Read the model definition and answer for the solid it produces. Units are mm, in the model's axes. A direction names the side the tool comes from. Coordinates: 2 decimals unless noted, no trailing zeros. Order: outer loops, then holes, each group sorted by start corner. A loop starts at its lowest first (then second) coordinate and runs counter-clockwise, first axis right, second up. Notation, with made-up numbers: (64.5, 21.25) -> (95.5, 21.25) arc R10 cw to (95.5, 35.25) -> close; hole circle Ø5 at (64.5, -34). An arc over 180 degrees is marked (long way). Answer in a Markdown table with one row per item.
from build123d import *

# Parameters (mm, degrees)
F1_DEPTH  = 6
F2_T      = -4
F3_DEPTH  = 25.4
F4_W      = 10.761987894
F4_H      = 6
F4_H_2    = 27.5
F5_DEPTH  = 4
F6_W      = 10.761987894
F6_H      = 6
F6_H_2    = 27.5
F7_DEPTH  = 4
F9_DEPTH  = 50
F10_DEPTH = 50
F11_DEPTH = 50
F12_DEPTH = 1
F13_DEPTH = 1
F14_DEPTH = 1
F15_DEPTH = 1
F18_DEPTH = 4
F20_DEPTH = 9
F21_R     = 1.5
F22_DEPTH = 7
F23_R     = 1.5
F24_DEPTH = 7
F25_R     = 1.5
F26_DEPTH = 7
F27_R     = 1.5
F28_DEPTH = 7
F29_R     = 7.5
F30_DEPTH = 25.4


with BuildPart() as f1:
    # F0 (on Top) → F1 (new body)
    with BuildSketch(Plane.XY):
        with BuildLine():
            Line((6.0000014261, 20.4372135154), (1.4261e-06, 20.4372135154))
            Line((1.4261e-06, 20.4372135154), (-5.9999985739, 20.4372135154))
            ThreePointArc((-5.9999985739, 20.4372135154), (-14.7648216341, 15.2020365756), (-19.9999985739, 6.4372135154))
            Line((-19.9999985739, 6.4372135154), (-19.9999985739, 0.4372135154))
            Line((-19.9999985739, 0.4372135154), (-19.9999985739, -5.5627864846))
            ThreePointArc((-19.9999985739, -5.5627864846), (-14.7648216341, -14.3276095448), (-5.9999985739, -19.5627864846))
            Line((-5.9999985739, -19.5627864846), (1.4261e-06, -19.5627864846))
            Line((1.4261e-06, -19.5627864846), (6.0000014261, -19.5627864846))
            ThreePointArc((6.0000014261, -19.5627864846), (14.7648244863, -14.3276095448), (20.0000014261, -5.5627864846))
            Line((20.0000014261, -5.5627864846), (20.0000014261, 6.4372135154))
            ThreePointArc((20.0000014261, 6.4372135154), (14.7648244863, 15.2020365756), (6.0000014261, 20.4372135154))
        make_face()
    extrude(amount=F1_DEPTH)

    # F2
    f2_openings = [f1.faces().sort_by_distance(p)[0] for p in [
        (1e-06, 0.437214, 6),
    ]]
    offset(amount=F2_T, openings=f2_openings)

    # F3 (cut): a face of the model
    f3_faces = [f1.faces().sort_by_distance(p)[0] for p in [
        (1.4261e-06, 0.4372135154, 4),
    ]]
    extrude(f3_faces, amount=-F3_DEPTH, mode=Mode.SUBTRACT)

    # F4 (on face) → F5 (join)
    with BuildSketch(Plane(origin=(16.0000014261, 0, 0), x_dir=(0, -1, 0), z_dir=(-1, 0, 0))):
        with Locations((-0.4372135154, 3)):
            Rectangle(F4_W, F4_H)
        with Locations((-0.4372135154, 19.75)):
            Rectangle(F4_W, F4_H_2)
    extrude(amount=-F5_DEPTH)

    # F6 (on face) → F7 (join)
    with BuildSketch(Plane.YZ.offset(-15.9999985739)):
        with Locations((0.4372135154, 3)):
            Rectangle(F6_W, F6_H)
        with Locations((0.4372135154, 19.75)):
            Rectangle(F6_W, F6_H_2)
    extrude(amount=-F7_DEPTH)

    # F8 (on face) → F9 (cut)
    with BuildSketch(Plane(origin=(-19.9999985739, 0, 0), x_dir=(0, -1, 0), z_dir=(-1, 0, 0))):
        with BuildLine():
            Line((-5.8182074624, 33.5), (-5.8182074624, 28.852354537))
            ThreePointArc((-5.8182074624, 28.852354537), (-3.9923402433, 32.177236302), (-0.4372135154, 33.5))
            Line((-0.4372135154, 33.5), (-5.8182074624, 33.5))
        make_face()
    extrude(amount=-F9_DEPTH, mode=Mode.SUBTRACT)

    # F8 (on face) → F10 (cut)
    with BuildSketch(Plane(origin=(-19.9999985739, 0, 0), x_dir=(0, -1, 0), z_dir=(-1, 0, 0))):
        with BuildLine():
            ThreePointArc((-0.4372135154, 33.5), (3.1179132125, 32.177236302), (4.9437804316, 28.852354537))
            Line((4.9437804316, 28.852354537), (4.9437804316, 33.5))
            Line((4.9437804316, 33.5), (-0.4372135154, 33.5))
        make_face()
    extrude(amount=-F10_DEPTH, mode=Mode.SUBTRACT)

    # F8 (on face) → F11 (cut)
    with BuildSketch(Plane(origin=(-19.9999985739, 0, 0), x_dir=(0, -1, 0), z_dir=(-1, 0, 0))):
        with BuildLine():
            ThreePointArc((3.8905718212, 24.7670060502), (4.0195248668, 25.3775186809), (4.0627864846, 26))
            ThreePointArc((4.0627864846, 26), (-1.0596948345, 30.4567383822), (-4.764998852, 24.7670060502))
            ThreePointArc((-4.764998852, 24.7670060502), (-0.4372135154, 21.5), (3.8905718212, 24.7670060502))
        make_face()
    extrude(amount=-F11_DEPTH, mode=Mode.SUBTRACT)

    # F12 (add): a face of the model
    f12_faces = [f1.faces().sort_by_distance(p)[0] for p in [
        (-17.9999985739, 5.8182074624, 17.4261772685),
    ]]
    extrude(f12_faces, amount=F12_DEPTH)

    # F13 (add): a face of the model
    f13_faces = [f1.faces().sort_by_distance(p)[0] for p in [
        (-17.9999985739, -4.9437804316, 17.4261772685),
    ]]
    extrude(f13_faces, amount=F13_DEPTH)

    # F14 (add): a face of the model
    f14_faces = [f1.faces().sort_by_distance(p)[0] for p in [
        (18.0000014261, 5.8182074624, 17.4261772685),
    ]]
    extrude(f14_faces, amount=F14_DEPTH)

    # F15 (add): a face of the model
    f15_faces = [f1.faces().sort_by_distance(p)[0] for p in [
        (18.0000014261, -4.9437804316, 17.4261772685),
    ]]
    extrude(f15_faces, amount=F15_DEPTH)

    # F17 (on face) → F18 (join)
    with BuildSketch(Plane(origin=(0, 0, 0), x_dir=(1, 0, 0), z_dir=(0, 0, -1))):
        with BuildLine():
            Line((1.4261e-06, 15.5627864846), (1.4261e-06, -0.4372135154))
            Line((1.4261e-06, -0.4372135154), (16.0000014261, -0.4372135154))
            Line((16.0000014261, -0.4372135154), (16.0000014261, 4.9437804316))
            ThreePointArc((16.0000014261, 4.9437804316), (11.9363973616, 11.4991824201), (5.3809953731, 15.5627864846))
            Line((5.3809953731, 15.5627864846), (1.4261e-06, 15.5627864846))
        make_face()
        with BuildLine():
            Line((-15.9999985739, 4.9437804316), (-15.9999985739, -0.4372135154))
            Line((-15.9999985739, -0.4372135154), (1.4261e-06, -0.4372135154))
            Line((1.4261e-06, -0.4372135154), (1.4261e-06, 15.5627864846))
            Line((1.4261e-06, 15.5627864846), (-5.3809925209, 15.5627864846))
            ThreePointArc((-5.3809925209, 15.5627864846), (-11.9363945094, 11.4991824201), (-15.9999985739, 4.9437804316))
        make_face()
        with BuildLine():
            Line((1.4261e-06, -0.4372135154), (-15.9999985739, -0.4372135154))
            Line((-15.9999985739, -0.4372135154), (-15.9999985739, -5.8182074624))
            ThreePointArc((-15.9999985739, -5.8182074624), (-11.9363945094, -12.3736094509), (-5.3809925209, -16.4372135154))
            Line((-5.3809925209, -16.4372135154), (1.4261e-06, -16.4372135154))
            Line((1.4261e-06, -16.4372135154), (1.4261e-06, -0.4372135154))
        make_face()
        with BuildLine():
            Line((16.0000014261, -0.4372135154), (1.4261e-06, -0.4372135154))
            Line((1.4261e-06, -0.4372135154), (1.4261e-06, -16.4372135154))
            Line((1.4261e-06, -16.4372135154), (5.3809953731, -16.4372135154))
            ThreePointArc((5.3809953731, -16.4372135154), (11.9363973616, -12.3736094509), (16.0000014261, -5.8182074624))
            Line((16.0000014261, -5.8182074624), (16.0000014261, -0.4372135154))
        make_face()
    extrude(amount=-F18_DEPTH)

    # F19 (on face) → F20 (join)
    with BuildSketch(Plane(origin=(0, 0, 0), x_dir=(1, 0, 0), z_dir=(0, 0, -1))):
        with BuildLine():
            Line((6, 31), (0, 31))
            Line((0, 31), (-6, 31))
            ThreePointArc((-6, 31), (-22.3271135618, 22.3271135618), (-31, 6))
            Line((-31, 6), (-31, -6))
            ThreePointArc((-31, -6), (-22.3271135618, -22.3271135618), (-6, -31))
            Line((-6, -31), (6, -31))
            ThreePointArc((6, -31), (22.3271135618, -22.3271135618), (31, -6))
            Line((31, -6), (31, 0))
            Line((31, 0), (31, 6))
            ThreePointArc((31, 6), (22.3271135618, 22.3271135618), (6, 31))
        make_face()
    extrude(amount=F20_DEPTH)

    # F21 (on face) → F22 (cut)
    with BuildSketch(Plane.XZ.offset(31)):
        with Locations((0, -4.4999574302)):
            Circle(F21_R)
    extrude(amount=-F22_DEPTH, mode=Mode.SUBTRACT)

    # F23 (on face) → F24 (cut)
    with BuildSketch(Plane(origin=(0, 31, 0), x_dir=(-1, 0, 0), z_dir=(0, 1, 0))):
        with Locations((0, -4.5)):
            Circle(F23_R)
    extrude(amount=-F24_DEPTH, mode=Mode.SUBTRACT)

    # F25 (on face) → F26 (cut)
    with BuildSketch(Plane.YZ.offset(31)):
        with Locations((-3.5, -4.5)):
            Circle(F25_R)
        with Locations((3.5, -4.5)):
            Circle(F25_R)
    extrude(amount=-F26_DEPTH, mode=Mode.SUBTRACT)

    # F27 (on face) → F28 (cut)
    with BuildSketch(Plane(origin=(-31, 0, 0), x_dir=(0, -1, 0), z_dir=(-1, 0, 0))):
        with Locations((-3.5, -4.5)):
            Circle(F27_R)
        with Locations((3.5, -4.5)):
            Circle(F27_R)
    extrude(amount=-F28_DEPTH, mode=Mode.SUBTRACT)

    # F29 (on face) → F30 (cut)
    with BuildSketch(Plane.XY.offset(4)):
        Circle(F29_R)
    extrude(amount=-F30_DEPTH, mode=Mode.SUBTRACT)


solid = f1.part
Q1. Consider line 1 (Z direction, x = 29, y = 3.5); line 2 (Y direction, x = 26, z = -4); line 3 (Z direction, x = 14.5, y = 9). Determine where each line is inside the solid, lowest interval first.
Outcome:
| item | result |
|---|---|
| line 1 | -9 to -6, -3 to 0 |
| line 2 | -17.92 to -4.91, -2.09 to 2.09, 4.91 to 17.92 |
| line 3 | -9 to 4 |
Q2. The part is cut by section D-D (z = 2). Write down the section's boundary in (x, y).
Outcome:
| item | result |
|---|---|
| outline | (-20, -5.56) arc R20.88 ccw to (-6, -19.56) -> (6, -19.56) arc R20.88 ccw to (20, -5.56) -> (20, 6.44) arc R20.88 ccw to (6, 20.44) -> (-6, 20.44) arc R20.88 ccw to (-20, 6.44) -> close; hole circle Ø15 at (0, 0) |
Q3. The part is cut by section A-A (x = 4.5). Write down the section's boundary in (y, z).
Outcome:
| item | result |
|---|---|
| outline | (-31, -9) -> (-6, -9) -> (-6, 4) -> (-15.56, 4) -> (-15.56, 6) -> (-19.56, 6) -> (-19.56, 0) -> (-31, 0) -> close; (6, -9) -> (31, -9) -> (31, 0) -> (20.44, 0) -> (20.44, 6) -> (16.44, 6) -> (16.44, 4) -> (6, 4) -> close |
Q4. For faces 4 (the face through (-27.55, 2.07, -4.05)), 5 (the face through (0, 16.437, 5)), 6 (the face through (0, -24, -4)), determine the directions among +Z, -Z, +X, -X, +Y, -Y from which every point of the face is accessible in a straight line to the end or side of a thin tool.
Outcome:
| item | result |
|---|---|
| face 4 | -X |
| face 5 | +Z |
| face 6 | -Y |
Q5. Given pin 1 (1.1 mm diameter, centred on x = -18, y = 6.5, fed in from +Z); pin 2 (1 mm diameter, centred on x = 1.5, z = 5, fed in from +Y); pin 3 (14.5 mm diameter, centred on y = 0.44, z = 26, fed in from -X); pin 4 (4 mm diameter, centred on y = 0.5, z = 25.5, fed in from +X), each flat-ended and moving along its own axis, determine where each tip first touches the part or whether it passes through.
Outcome:
| item | result |
|---|---|
| pin 1 | z = 28.85 |
| pin 2 | y = 20.44 |
| pin 3 | x = -20 |
| pin 4 | through |
Q6. For a pull along X with two mould halves and no side action, classify faces 1 (the face through (11.86, 12.45, 5.01)), 2 (the face through (27.55, 4.93, -4.05)), 3 (the face through (-22.14, -22.51, -4.44)) as pulls with the +X half, pulls with the -X half, needs draft (parallel to the pull), parting line crosses it, or undercut.
Outcome:
| item | result |
|---|---|
| face 1 | undercut |
| face 2 | needs draft |
| face 3 | pulls with the -X half |
Q7. The part is cut by section B-B (y = 3.5). Give the number of separate pieces and of enclosed holes in the cut face, then the cut area to 3 significant figures.
Outcome:
| item | result |
|---|---|
| separate pieces | 4 |
| enclosed holes | 0 |
| area | 679 mm² |
Q8. The part is cut by section C-C (z = 11.5). Write down the section's boundary in (x, y), then the cut area to 3 significant figures.
Outcome:
| item | result |
|---|---|
| outline | (-20, -5.94) -> (-16, -5.94) -> (-16, 6.82) -> (-20, 6.82) -> close; (16, -5.94) -> (20, -5.94) -> (20, 6.82) -> (16, 6.82) -> close |
| area | 102 mm² |
